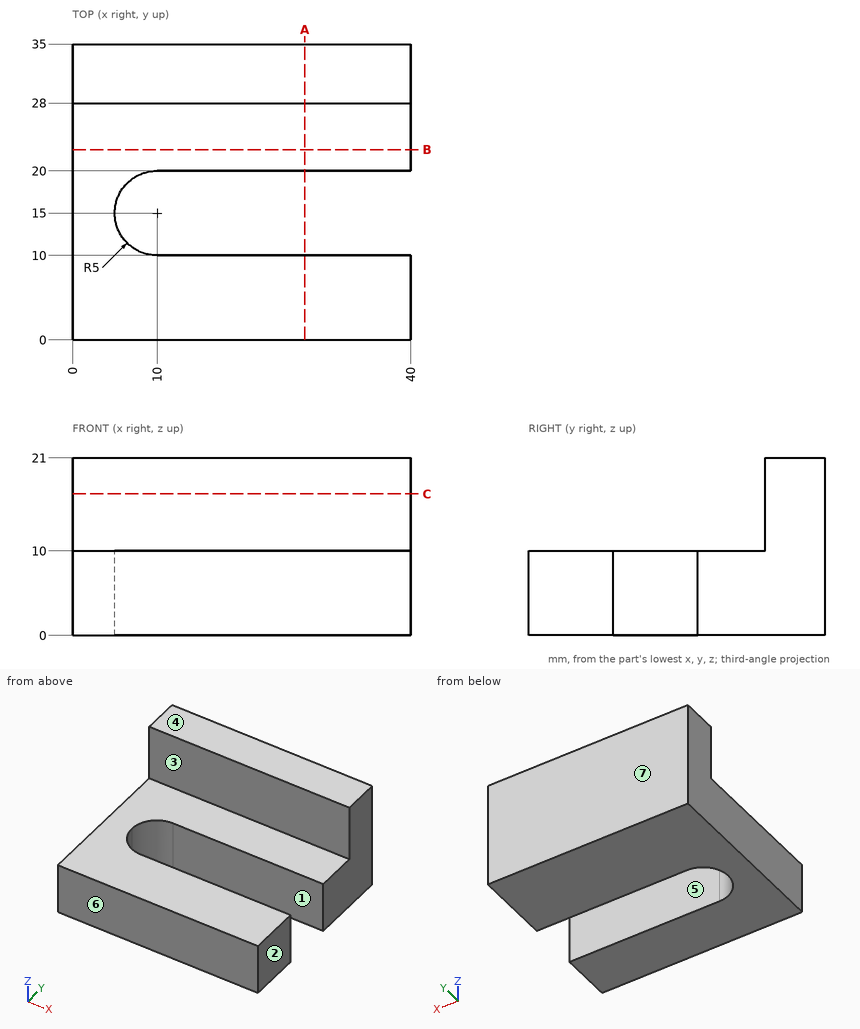
Design review of the part shown in the three views and the two pictorial views. Dimensions are in mm from the part's minimum x, y and z. A direction names the side the tool comes from. Round coordinates to 2 decimals unless told otherwise and drop trailing zeros. Write each loop counter-clockwise with the first axis right and the second up, starting at its lowest first coordinate (ties: lowest second). Pieces come first, ordered by that corner, then holes. Notation, with made-up numbers: (7, 42.5) - (17, 42.5) arc R23 cw to (17, 52.5) - close; hole circle Ø10 at (88.25, 32). An arc over 180 degrees is marked (long way). Write item = value, one per line. Start each with the question number.
1. Consider section A-A on x = 27.5. State the section outline as (y, z) points, plus the area to 3 significant figures.
2. Consider section B-B on y = 22.5. State the section outline as (x, z) points.
3. Consider section C-C on z = 16.75. State the section outline as (x, y) points.
4. Draft analysis for pull direction Y (two halves, no side actions). For the marked faces 4, 5, 6 and 7, state which applies: released by +Y, released by -Y, zero draft, split by the parting line, or undercut.
5. Wall thickness on L1, parallel to Y at x = 35, z = 2; L2, parallel to Z at x = 19, y = 26; L3, parallel to Y at x = 37, z = 11.25: over which ranges is each line inside the solid? List them lowest first.
6. For pin 1 Ø10 at (y, z) = (16.5, 12.5) entering from -X; pin 2 Ø2 at (x, y) = (11, 25) entering from +Z; pin 3 Ø3.5 at (x, z) = (16.5, 14.5) entering from -Y, all flat-tipped, find the tip position at first contact; note any pin that passes through.
7. For the marked faces 1, 2 and 3, list the 3-axis set-ups (+Z, -Z, +X, -X, +Y, -Y) from which the entire face can be reached by the end or side of a thin tool; tool diameter is ignored.
Evaluation:
q1.outline = (0, 0) - (10, 0) - (10, 10) - (0, 10) - close; (20, 0) - (35, 0) - (35, 21) - (28, 21) - (28, 10) - (20, 10) - close
q1.area = 327 mm2
q2.outline = (0, 0) - (40, 0) - (40, 10) - (0, 10) - close
q3.outline = (0, 28) - (40, 28) - (40, 35) - (0, 35) - close
q4.face_4 = zero draft
q4.face_5 = undercut
q4.face_6 = released by -Y
q4.face_7 = released by +Y
q5.L1 = 0 to 10, 20 to 35
q5.L2 = 0 to 10
q5.L3 = 28 to 35
q6.pin_1 = 0
q6.pin_2 = 10
q6.pin_3 = 28
q7.face_1 = +Z, -Z, +X
q7.face_2 = +Z, -Z, +X, +Y, -Y
q7.face_3 = +Z, +X, -X, -Y
